Check sheet for the drawn part. Datum: minimum x, y, z corner. Units: mm. A direction names the side the tool comes from. Round coordinates to 2 decimals unless told otherwise and drop trailing zeros. Order: outer loops, then holes, each group sorted by start corner. A loop starts at its lowest first (then second) coordinate and runs counter-clockwise, first axis right, second up. Notation, with made-up numbers: (79.25, 17) -> (122.25, 17) arc R24 cw to (122.25, 54) -> close; hole circle Ø5 at (82.25, -40). An arc over 180 degrees is marked (long way). Answer as a JSON object with one key per item and string values. Group by question number.
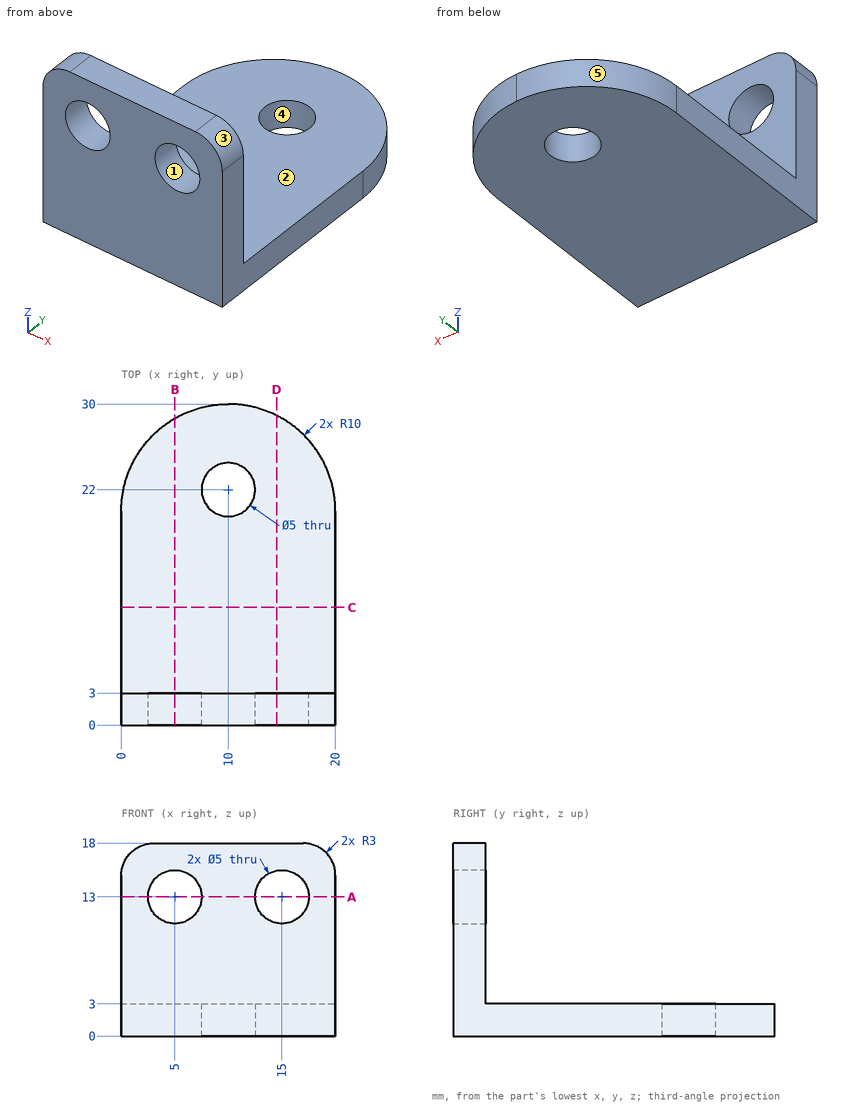
Item 1: Sectioned sample at C-C, the plane y = 11. Enter the section's corners in (x, z).
Item 2: Mould release check, pull along Y, two halves, no side actions. Record for the marked faces 3, 4 and 5: pulls with the +Y half, pulls with the -Y half, needs draft (parallel to the pull), parting line crosses it, or undercut.
Item 3: Set-up check for the marked faces 1 and 2: record each of +Z, -Z, +X, -X, +Y, -Y from which the full face is reachable in a straight line by a thin tool's end or side.
Item 4: Depth check by flat-ended pin: pin 1 Ø4 at (x, z) = (15, 13) entering from -Y; pin 2 Ø4 at (x, z) = (6, 15) entering from +Y; pin 3 Ø10 at (x, y) = (12.5, 15) entering from +Z. Enter the tip coordinate at first touch or a pass-through.
Item 5: Sectioned sample at A-A, the plane z = 13. Enter the section's corners in (x, y), then the cut area to 3 significant figures.
Item 6: Thickness scan on L1, parallel to X at y = 0.9, z = 13; L2, parallel to Z at x = 16, y = 26; L3, parallel to Y at x = 10, z = 1.6. Record the ranges inside material, lowest first.
Item 7: Sectioned sample at D-D, the plane x = 14.5. Enter the section's corners in (y, z), then the cut area to 3 significant figures.
Item 8: Sectioned sample at B-B, the plane x = 5. Enter the section's corners in (y, z).
Result:
{
 "1": {"outline": "(0, 0) -> (20, 0) -> (20, 3) -> (0, 3) -> close"},
 "2": {"face 3": "needs draft", "face 4": "undercut", "face 5": "pulls with the +Y half"},
 "3": {"face 1": "+Y, -Y", "face 2": "+Z, +X, -X, +Y"},
 "4": {"pin 1": "passes through", "pin 2": "stops at y = 3", "pin 3": "stops at z = 3"},
 "5": {"outline": "(0, 0) -> (2.5, 0) -> (2.5, 3) -> (0, 3) -> close; (7.5, 0) -> (12.5, 0) -> (12.5, 3) -> (7.5, 3) -> close; (17.5, 0) -> (20, 0) -> (20, 3) -> (17.5, 3) -> close", "area": "30.0 mm2"},
 "6": {"L1": "x = 0 to 2.5, 7.5 to 12.5, 17.5 to 20", "L2": "z = 0 to 3", "L3": "y = 0 to 19.5, 24.5 to 30"},
 "7": {"outline": "(0, 0) -> (28.93, 0) -> (28.93, 3) -> (3, 3) -> (3, 10.55) -> (0, 10.55) -> close; (0, 15.45) -> (3, 15.45) -> (3, 18) -> (0, 18) -> close", "area": "117 mm2"},
 "8": {"outline": "(0, 0) -> (28.66, 0) -> (28.66, 3) -> (3, 3) -> (3, 10.5) -> (0, 10.5) -> close; (0, 15.5) -> (3, 15.5) -> (3, 18) -> (0, 18) -> close"}
}
